from build123d import *

# Parameters (mm, degrees)
CIRPATTERN1_COUNT  = 3
CUT_EXTRUDE1_START = 6
CUT_EXTRUDE1_DEPTH = 2.5
ECHELLE1_SCALE     = 2
ECHELLE2_SCALE     = 0.25


with BuildPart() as part:
    # Sketch1 → Revolve3 (revolve)
    with BuildSketch(Plane.XY, mode=Mode.PRIVATE) as revolve3_sk:
        Polygon((0, 0), (0, 5), (1, 6), (19, 6), (19, 7.5), (20.4, 7.5), (20.4, 7.15), (21.5, 7.15), (21.5, 7.5), (46, 7.5), (46, 10), (46.5, 10), (46.5, 20), (53.5, 20), (53.5, 0), align=None)
    revolve(revolve3_sk.sketch.rotate(Axis((0, 0, 0), (1, 0, 0)), 180), axis=Axis((0, 0, 0), (1, 0, 0)))

    # Sketch3 → 4.0 _4_ Diameter Hole1 (revolve, cut)
    with BuildSketch(Plane(origin=(53.5, 16.25, 0), x_dir=(0, 0, -1), z_dir=(0, 1, 0))):
        Polygon((0, 0), (0, 13.201721238), (2, 12), (2, 0), align=None)
    f_4_0_4_diameter_hole1 = revolve(axis=Axis((59.85, 16.25, 0), (-1, 0, 0)), mode=Mode.SUBTRACT)

    # CirPattern1: 4.0 _4_ Diameter Hole1 ×3 about axis
    cirpattern1_axis = Axis((0, 0, 0), (1, 0, 0))
    for i in range(1, CIRPATTERN1_COUNT):
        add(f_4_0_4_diameter_hole1.rotate(cirpattern1_axis, i * 360 / CIRPATTERN1_COUNT), mode=Mode.SUBTRACT)

    # Sketch6 → Cut-Extrude1 (cut)
    with BuildSketch(Plane(origin=(0, 0, 0), x_dir=(1, 0, 0), z_dir=(0, 1, 0)).offset(CUT_EXTRUDE1_START)):
        with BuildLine():
            Line((4.5, -2), (14.5, -2))
            ThreePointArc((14.5, -2), (16.5, 0), (14.5, 2))
            Line((14.5, 2), (4.5, 2))
            ThreePointArc((4.5, 2), (2.5, 0), (4.5, -2))
        make_face()
    extrude(amount=-CUT_EXTRUDE1_DEPTH, mode=Mode.SUBTRACT)


with BuildPart() as part_1:
    # Echelle1: scaled about (39.34390125, -0.03827419, -1e-09)
    add(part.part.scale(ECHELLE1_SCALE).moved(Location((-39.34390125, 0.03827419, 1e-09))))


with BuildPart() as part_2:
    # Echelle2: scaled about (39.34390125, -0.03827419, -1e-09)
    add(part_1.part.scale(ECHELLE2_SCALE).moved(Location((29.507925938, -0.028705642, -1e-09))))


solid = part_2.part
Part model, mm, in its own coordinate system. A direction names the side the tool comes from. Coordinates: 2 decimals unless noted, no trailing zeros. Loops run counter-clockwise (first coordinate to the right, second up) from the corner with the lowest first, then second, coordinate; pieces in that order, holes last. Notation, with made-up numbers: M -32,47.25 L -4,47.25 A28 ccw -4,83.25 Z; hole C 29,46 d10. An arc over 180 degrees is marked long. Use a Markdown table: item, result. Add a question column.
Q1. Mould opens along Z. For faces 1 (the flat face through (19.672, 0, 0)), 2 (the cylindrical face through (30.2, 2.8, 2.2)), 3 (the flat face through (24, 2, 1)) say: +Z half, -Z half, draft (parallel to the pull), parting line (faces both ways), or undercut.
Q2. Which spindle directions (+Z, -Z, +X, -X, +Y, -Y) get a long thin tool onto all of the face, cutting with end or side? Do faces 4 (the cylindrical face through (27.92, 2.36, 0.02)), 5 (the flat face through (46.422, 0, 0)), 6 (the cylindrical face through (24.73, -2.88, -0.9)). Say none if no direction does.
Q3. Cut at B-B (y = -6). Write the cut outline in (x, z), and give its area (3 significant figures).
Q4. Probe L1, parallel to Y at x = 44.7, z = 0; L2, parallel to X at y = -6.75, z = -6.75; L3, parallel to X at y = -3.25, z = 1.25. List the from-to ranges inside material, lowest first.
Q5. Pin check, flat tips, straight feed: P1, Ø4, axis at x = 23, z = 4, coming from the +Y side; P2, Ø0.6, axis at x = 23, z = 0, coming from the +Y side; P3, Ø2, axis at x = 27.5, z = -3.5, coming from the -Y side; P4, Ø1.8, axis at y = -4.08, z = 7.04, coming from the -X side. Stop position of each tip, or through.
Worked out:
| question | item | result |
|---|---|---|
| 1 | face 1 | draft |
| 1 | face 2 | parting line |
| 1 | face 3 | undercut |
| 2 | face 4 | +Y |
| 2 | face 5 | +Z, -Z, +X, +Y, -Y |
| 2 | face 6 | -X |
| 3 | outline | M 42.92,-8.01 L 46.42,-8.01 L 46.42,8.01 L 42.92,8.01 Z |
| 3 | area | 56.1 mm2 |
| 4 | L1 | y = -10.02 to 7.11, 9.11 to 9.98 |
| 4 | L2 | x = 42.92 to 46.42 |
| 4 | L3 | x = 29.17 to 46.42 |
| 5 | P1 | stops at y = 2.22 |
| 5 | P2 | stops at y = 1.73 |
| 5 | P3 | stops at y = -1.68 |
| 5 | P4 | passes through |
